Check sheet for the modelled part. Datum: model origin and axes. Units: mm. A direction names the side the tool comes from. Give positions to 0.01 mm unless a question says otherwise; leave off trailing zeros. Write each loop counter-clockwise with the first axis right and the second up, starting at its lowest first coordinate (ties: lowest second). Pieces come first, ordered by that corner, then holes. Notation, with made-up numbers: M -21,27.5 L 6,27.5 A35 ccw 6,60.5 Z; hole C 61.5,76 d9. An arc over 180 degrees is marked long. One line per item, written item: value. Start each with the question number.
from build123d import *

# Parameters (mm, degrees)
F0_R     = 1.5
F0_W     = 7
F0_H     = 6
F1_DEPTH = 1.5
F2_DEPTH = 7.5
F3_R     = 1.4
F4_DEPTH = 25
F5_R     = 2.99999


# Not quite as in the source:
# - a fillet or chamfer is up to 0.001 mm smaller than in the source, because OpenCascade refuses the exact size


with BuildPart() as f1:
    # F0 (on Top) → F1 (new body)
    with BuildSketch(Plane.XY):
        with BuildLine():
            add(Edge.make_bspline(
                [(-5.5561550838, 5.6573497621), (-4.0955413133, 3.5522743128), (-3.2797986642, 3.3143495675), (0, 3.173440462)],
                knots=[0, 0, 0, 0, 6.0861042323, 6.0861042323, 6.0861042323, 6.0861042323], degree=3))
            ThreePointArc((-5.5561550838, 5.6573497621), (-11.1647533144, 9.6698318912), (-7.2436210565, 3.9969923231))
            add(Edge.make_bspline(
                [(-7.2436210565, 3.9969923231), (-6.2028751709, 2.9064782429), (-5.828993395, 2.9744568747), (-5.7950043119, 0)],
                knots=[0, 0, 0, 0, 4.2514042508, 4.2514042508, 4.2514042508, 4.2514042508], degree=3))
            add(Edge.make_bspline(
                [(-7.2436210565, -3.9969923231), (-6.2028751709, -2.9064782429), (-5.828993395, -2.9744568747), (-5.7950043119, 0)],
                knots=[0, 0, 0, 0, 4.2514042508, 4.2514042508, 4.2514042508, 4.2514042508], degree=3))
            ThreePointArc((-7.2436210565, -3.9969923231), (-11.1647533144, -9.6698318912), (-5.5561550838, -5.6573497621))
            add(Edge.make_bspline(
                [(-5.5561550838, -5.6573497621), (-4.0955413133, -3.5522743128), (-3.2797986642, -3.3143495675), (0, -3.173440462)],
                knots=[0, 0, 0, 0, 6.0861042323, 6.0861042323, 6.0861042323, 6.0861042323], degree=3))
            add(Edge.make_bspline(
                [(5.5561550838, -5.6573497621), (4.0955413133, -3.5522743128), (3.2797986642, -3.3143495675), (0, -3.173440462)],
                knots=[0, 0, 0, 0, 6.0861042323, 6.0861042323, 6.0861042323, 6.0861042323], degree=3))
            ThreePointArc((5.5561550838, -5.6573497621), (11.1647533144, -9.6698318912), (7.2436210565, -3.9969923231))
            add(Edge.make_bspline(
                [(7.2436210565, -3.9969923231), (6.2028751709, -2.9064782429), (5.828993395, -2.9744568747), (5.7950043119, 0)],
                knots=[0, 0, 0, 0, 4.2514042508, 4.2514042508, 4.2514042508, 4.2514042508], degree=3))
            add(Edge.make_bspline(
                [(7.2436210565, 3.9969923231), (6.2028751709, 2.9064782429), (5.828993395, 2.9744568747), (5.7950043119, 0)],
                knots=[0, 0, 0, 0, 4.2514042508, 4.2514042508, 4.2514042508, 4.2514042508], degree=3))
            ThreePointArc((7.2436210565, 3.9969923231), (11.1647533144, 9.6698318912), (5.5561550838, 5.6573497621))
            add(Edge.make_bspline(
                [(5.5561550838, 5.6573497621), (4.0955413133, 3.5522743128), (3.2797986642, 3.3143495675), (0, 3.173440462)],
                knots=[0, 0, 0, 0, 6.0861042323, 6.0861042323, 6.0861042323, 6.0861042323], degree=3))
        make_face()
        with Locations((-8.71, -7.175)):
            Circle(F0_R, mode=Mode.SUBTRACT)
        with Locations((8.71, -7.175)):
            Circle(F0_R, mode=Mode.SUBTRACT)
        with Locations((-8.71, 7.175)):
            Circle(F0_R, mode=Mode.SUBTRACT)
        Rectangle(F0_W, F0_H, mode=Mode.SUBTRACT)
        with Locations((8.71, 7.175)):
            Circle(F0_R, mode=Mode.SUBTRACT)
    extrude(amount=F1_DEPTH)

    # F0 (on Top) → F2 (join)
    with BuildSketch(Plane.XY):
        Rectangle(F0_W, F0_H)
    extrude(amount=F2_DEPTH)

    # F3 (on face) → F4 (cut)
    with BuildSketch(Plane(origin=(-3.5, 0, 0), x_dir=(0, -1, 0), z_dir=(-1, 0, 0))):
        with Locations((0, 4.8)):
            Circle(F3_R)
    extrude(amount=-F4_DEPTH, mode=Mode.SUBTRACT)

    # F5 (radius 3 in the source; OpenCascade refuses exactly that, so slightly less here)
    f5_edges = [f1.edges().sort_by_distance(p)[0] for p in [
        (0, 3, 7.5),
        (0, -3, 7.5),
    ]]
    fillet(f5_edges, radius=F5_R)


solid = f1.part
1) Cross-section at B-B (y = -6.75). Record the boundary of the cut face in (x, z).
2) Material ranges on L1, parallel to Y at x = 8.71, z = 1.05 (3 decimals); L2, parallel to Z at x = 7.25, y = -9.75; L3, parallel to X at y = -1, z = 3.75, recorded low to high. Write a range as from..to.
3) Cross-section at A-A (x = 8.71). Record the boundary of the cut face in (y, z) (3 decimals).
4) Tool access check on faces 5 (the flat face through (0, 3, 3)), 6 (the cylindrical face through (10.096, -7.75, 0.74)), 7 (the flat face through (3.5, 0, 3)). Record the directions out of +Z, -Z, +X, -X, +Y, -Y that give a thin tool (end or side, any length) a straight path to the whole face; none if there is none.
5) Draft check along X on faces 1 (the flat face through (-3.5, 0, 3)), 2 (the cylindrical face through (11.26, 9.57, 0.74)), 3 (the cylindrical face through (9.516, 8.44, 0.74)), 4 (the flat face through (0, -3, 3)). Enter one of: released by +X, released by -X, zero draft, split by the parting line, or undercut.
6) Gauge pin test, flat ends, axial feed: pin 1 (2 mm diameter, centred on x = -3.5, z = 3, fed in from -Y); pin 2 (4 mm diameter, centred on x = -8.71, y = 7.175, fed in from +Z); pin 3 (3.5 mm diameter, centred on x = -1, z = 2.5, fed in from -Y). Record the tip position at first contact, or that the pin passes through.
7) Cross-section at C-C (z = 4.8). Record the boundary of the cut face in (x, y), plus the area to 3 significant figures.
8) Cross-section at D-D (z = 1). State how many separate pieces and enclosed holes the cut face has, plus the area to 3 significant figures.
Data:
1. outline: M -12.18,0 L -10.15,0 L -10.15,1.5 L -12.18,1.5 Z; M -7.27,0 L -5.24,0 L -5.24,1.5 L -7.27,1.5 Z; M 5.24,0 L 7.27,0 L 7.27,1.5 L 5.24,1.5 Z; M 10.15,0 L 12.18,0 L 12.18,1.5 L 10.15,1.5 Z
2. L1: y = -10.675..-8.675, -5.675..-3.675, 3.675..5.675, 8.675..10.675
2. L2: z = 0..1.5
2. L3: x = -3.5..3.5
3. outline: M -10.675,0 L -8.675,0 L -8.675,1.5 L -10.675,1.5 Z; M -5.675,0 L -3.675,0 L -3.675,1.5 L -5.675,1.5 Z; M 3.675,0 L 5.675,0 L 5.675,1.5 L 3.675,1.5 Z; M 8.675,0 L 10.675,0 L 10.675,1.5 L 8.675,1.5 Z
4. face 5: +Z, +X, -X, +Y
4. face 6: +Z, -Z
4. face 7: +Z, +X, +Y, -Y
5. face 1: released by -X
5. face 2: undercut
5. face 3: undercut
5. face 4: zero draft
6. pin 1: stops at y = -3
6. pin 2: stops at z = 1.5
6. pin 3: stops at y = -3.39
7. outline: M -3.5,-2.98 L 3.5,-2.98 L 3.5,-1.4 L -3.5,-1.4 Z; M -3.5,1.4 L 3.5,1.4 L 3.5,2.98 L -3.5,2.98 Z
7. area: 22.2 mm2
8. separate pieces: 1
8. enclosed holes: 4
8. area: 223 mm2
